from build123d import *

# Parameters (mm, degrees)
F0_W      = 139.7
F0_H      = 55.88
F1_DEPTH  = 55.88
F2_W      = 101.6
F2_H      = 25.4
F3_DEPTH  = 55.881
F4_R      = 27.93999
F5_R      = 15.24
F6_DEPTH  = 55.881
F7_W      = 76.2
F7_H      = 25.4
F8_DEPTH  = 55.881
F9_R      = 15.24
F10_DEPTH = 55.881


# Not quite as in the source:
# - a fillet or chamfer is up to 0.001 mm smaller than in the source, because OpenCascade refuses the exact size


with BuildPart() as f1:
    # F0 (on Top) → F1 (new body)
    with BuildSketch(Plane.XY):
        with Locations((69.85, 27.94)):
            Rectangle(F0_W, F0_H)
    extrude(amount=F1_DEPTH)

    # F2 (on face) → F3 (cut, through all)
    with BuildSketch(Plane(origin=(0, 0, 0), x_dir=(1, 0, 0), z_dir=(0, 0, -1))):
        with Locations((137.16, -27.94)):
            Rectangle(F2_W, F2_H)
    extrude(amount=-F3_DEPTH, mode=Mode.SUBTRACT)

    # F4 (radius 27.94 in the source; OpenCascade refuses exactly that, so slightly less here)
    f4_edges = [f1.edges().sort_by_distance(p)[0] for p in [
        (139.7, 48.26, 55.88),
        (139.7, 7.62, 55.88),
        (139.7, 7.62, 0),
        (139.7, 48.26, 0),
        (0, 55.88, 27.94),
        (0, 0, 27.94),
    ]]
    fillet(f4_edges, radius=F4_R)

    # F5 (on face) → F6 (cut, through all)
    with BuildSketch(Plane(origin=(0, 55.88, 0), x_dir=(-1, 0, 0), z_dir=(0, 1, 0))):
        with Locations((-111.76, 27.94)):
            Circle(F5_R)
    extrude(amount=-F6_DEPTH, mode=Mode.SUBTRACT)

    # F7 (on face) → F8 (cut, through all)
    with BuildSketch(Plane(origin=(0, 55.88, 0), x_dir=(-1, 0, 0), z_dir=(0, 1, 0))):
        with Locations((-15.24, 27.94)):
            Rectangle(F7_W, F7_H)
    extrude(amount=-F8_DEPTH, mode=Mode.SUBTRACT)

    # F9 (on face) → F10 (cut, through all)
    with BuildSketch(Plane(origin=(0, 0, 0), x_dir=(1, 0, 0), z_dir=(0, 0, -1))):
        with Locations((27.94, -27.94)):
            Circle(F9_R)
    extrude(amount=-F10_DEPTH, mode=Mode.SUBTRACT)


solid = f1.part
Check sheet for the modelled part. Datum: model origin and axes. Units: mm. A direction names the side the tool comes from. Give positions to 0.01 mm unless a question says otherwise; leave off trailing zeros. Order: outer loops, then holes, each group sorted by start corner. A loop starts at its lowest first (then second) coordinate and runs counter-clockwise, first axis right, second up. Notation, with made-up numbers: (-29.75, 4) - (24.25, 4) arc R33 cw to (24.25, 42) - close; hole circle Ø2 at (38.25, 7). An arc over 180 degrees is marked (long way). Answer as CSV lines item,"result".
1. Section check B-B (y = 21). Record the boundary of the cut face in (x, z), then the cut area to 3 significant figures.
Result sheet:
outline,"(0.88, 0) - (14.37, 0) - (14.37, 15.24) - (0.88, 15.24) - close; (0.88, 40.64) - (14.37, 40.64) - (14.37, 55.88) - (0.88, 55.88) - close; (41.51, 0) - (86.36, 0) - (86.36, 55.88) - (41.51, 55.88) - (41.51, 40.64) - (53.34, 40.64) - (53.34, 15.24) - (41.51, 15.24) - close"
area,"2,620 mm²"
2. Section check C-C (x = 50.5). Record the boundary of the cut face in (y, z), then the cut area to 3 significant figures.
Result sheet:
outline,"(0, 0) - (55.88, 0) - (55.88, 15.24) - (0, 15.24) - close; (0, 40.64) - (55.88, 40.64) - (55.88, 55.88) - (0, 55.88) - close"
area,"1,700 mm²"
3. Tool access check on faces 4 (the face through (86.36, 28, 28)), 5 (the face through (131.3, 7.73, 47.91)), 6 (the face through (39, 16, 15.24)). Record the directions out of +Z, -Z, +X, -X, +Y, -Y that give a thin tool (end or side, any length) a straight path to the whole face; none if there is none.
Result sheet:
face 4,"+Z, -Z, +X"
face 5,"+Z, +X, +Y, -Y"
face 6,"-X, +Y, -Y"
4. Section check A-A (x = 102). Record the boundary of the cut face in (y, z), then the cut area to 3 significant figures.
Result sheet:
outline,"(0, 0) - (15.24, 0) - (15.24, 16.24) - (0, 16.24) - close; (0, 39.64) - (15.24, 39.64) - (15.24, 55.88) - (0, 55.88) - close; (40.64, 0) - (55.88, 0) - (55.88, 16.24) - (40.64, 16.24) - close; (40.64, 39.64) - (55.88, 39.64) - (55.88, 55.88) - (40.64, 55.88) - close"
area,"990 mm²"
5. Mould release check, pull along Y, two halves, no side actions. Record for faces 1 (the face through (55, 28, 0)), 2 (the face through (101, 40.64, 40)), 3 (the face through (7.97, 8.4, 48.37)): released by +Y, released by -Y, zero draft, split by the parting line, or undercut.
Result sheet:
face 1,"zero draft"
face 2,"undercut"
face 3,"released by -Y"
6. Scan lines: probe 1 along Y at (x, z) = (87, 18.5); probe 2 along X at (y, z) = (48, 27); probe 3 along Y at (x, z) = (27, 12). Record each from-to range of solid material in increasing order. Write a range as from..to.
Result sheet:
probe 1,"0..15.24, 40.64..55.88"
probe 2,"53.34..96.55, 126.97..139.68"
probe 3,"0.02..12.73, 43.15..55.86"
7. Go/stop test with flat-tipped pins: P1, Ø7.5, axis at y = 15, z = 28.5, coming from the -X side; P2, Ø1.5, axis at x = 17, z = 47, coming from the -Y side; P3, Ø1.5, axis at y = 18, z = 18, coming from the +X side. Record where each tip stops, or that it passes through.
Result sheet:
P1,"x = 53.34"
P2,"y = 1.92"
P3,"x = 86.36"
